```python
from build123d import *

# Parameters (mm, degrees)
SKETCH1_R          = 13.29266328
GEAR_BASE_DEPTH    = 2.921
GEAR_CUT_DEPTH     = 20.685496137
GEAR_TEETH_COUNT   = 10
SKETCH9_R          = 3.175
CUT_EXTRUDE2_DEPTH = 20.416099984


with BuildPart() as part:
    # Sketch1 → GEAR_BASE (new, symmetric)
    with BuildSketch(Plane.XY):
        Circle(SKETCH1_R)
    extrude(amount=GEAR_BASE_DEPTH, both=True)

    # Sketch2 → GEAR_CUT (cut, through all)
    with BuildSketch(Plane.XY.offset(2.921)):
        with BuildLine():
            ThreePointArc((-11.256508875, -7.070071076), (-12.642074031, -4.107658854), (-13.262390488, -0.896602257))
            ThreePointArc((-13.262390488, -0.896602257), (-12.138766836, -1.422314596), (-10.939670247, -1.740231168))
            ThreePointArc((-10.939670247, -1.740231168), (-9.896826282, -1.831227702), (-8.853265833, -1.748853585))
            ThreePointArc((-8.853265833, -1.748853585), (-8.313717175, -1.858972165), (-7.983334635, -2.299524357))
            ThreePointArc((-7.983334635, -2.299524357), (-7.90129627, -2.567286784), (-7.810279896, -2.832132079))
            ThreePointArc((-7.810279896, -2.832132079), (-7.818614904, -3.382740273), (-8.19039286, -3.78896682))
            ThreePointArc((-8.19039286, -3.78896682), (-9.083069289, -4.335714202), (-9.873261359, -5.022300247))
            ThreePointArc((-9.873261359, -5.022300247), (-10.656484205, -5.984311448), (-11.256508875, -7.070071076))
        make_face()
    gear_cut = extrude(amount=-GEAR_CUT_DEPTH, mode=Mode.SUBTRACT)

    # GEAR_TEETH: GEAR_CUT ×10 about axis
    gear_teeth_axis = Axis((0, 0, 0), (0, 0, 1))
    for i in range(1, GEAR_TEETH_COUNT):
        add(gear_cut.rotate(gear_teeth_axis, i * 360 / GEAR_TEETH_COUNT), mode=Mode.SUBTRACT)

    # Sketch9 → Cut-Extrude2 (cut, through all)
    with BuildSketch(Plane(origin=(0, 0, -2.921), x_dir=(-1, 0, 0), z_dir=(0, 0, -1))):
        Circle(SKETCH9_R)
        Polygon((1.998092242, -2.467438428), (3.143647563, -0.445089877), (5.165996114, -1.590645198), (4.020440792, -3.612993749), align=None)
    extrude(amount=-CUT_EXTRUDE2_DEPTH, mode=Mode.SUBTRACT)


solid = part.part
```
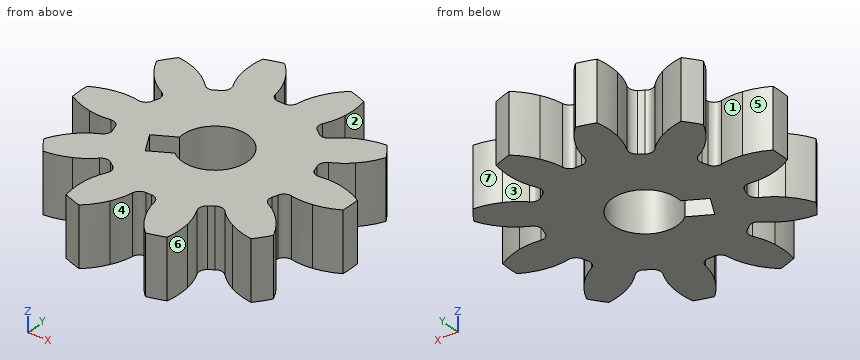
Geometry: final body of the model. Coordinates: model frame, mm. Face numbers are marked on the shaded views. A direction names the side the tool comes from. Round coordinates to 2 decimals unless told otherwise and drop trailing zeros. Loops run counter-clockwise (first coordinate to the right, second up) from the corner with the lowest first, then second, coordinate; pieces in that order, holes last.
Item 1: Section A-A, the plane y = 0. Output: boundary loops of the cut face in (x, z) (3 decimals).
Checked values:
outline: (-13.293, -2.921) - (-3.175, -2.921) - (-3.175, 2.921) - (-13.293, 2.921) - close; (3.175, -2.921) - (13.293, -2.921) - (13.293, 2.921) - (3.175, 2.921) - close
Item 2: Section B-B, the plane x = -7. Output: boundary loops of the cut face in (y, z).
Checked values:
outline: (-7.35, -2.92) - (7.35, -2.92) - (7.35, 2.92) - (-7.35, 2.92) - close
Item 3: Reachability of the marked faces 1, 2, 3 and 4 from +Z, -Z, +X, -X, +Y, -Y: full face, straight path, thin tool, end or side. Return the list, or none.
Checked values:
face 1: +Z, -Z
face 2: +Z, -Z, +X
face 3: +Z, -Z, +Y
face 4: +Z, -Z, -Y
Item 4: Line query: L1, parallel to Y at x = 0, z = 1.55 (3 decimals); L2, parallel to X at y = 0, z = -1.05 (3 decimals); L3, parallel to X at y = 0.5, z = 0.95. Output: solid intervals per line, ascending.
Checked values:
L1: y = -8.308 to -3.175, 3.175 to 8.308
L2: x = -13.293 to -3.175, 3.175 to 13.293
L3: x = -13.28 to -3.14, 3.14 to 13.28
Item 5: Section C-C, the plane x = 5.5. Output: boundary loops of the cut face in (y, z).
Checked values:
outline: (-6.39, -2.92) - (6.39, -2.92) - (6.39, 2.92) - (-6.39, 2.92) - close
Item 6: Mould query, pull axis X, two halves, no side actions, for the marked faces 5, 6 and 7. Classes: released by +X, released by -X, zero draft, split by the parting line, or undercut.
Checked values:
face 5: released by -X
face 6: released by +X
face 7: undercut
